Read the model definition and answer for the solid it produces. Units are mm, in the model's axes. Give positions to 0.01 mm unless a question says otherwise; leave off trailing zeros. Order: outer loops, then holes, each group sorted by start corner. A loop starts at its lowest first (then second) coordinate and runs counter-clockwise, first axis right, second up. Notation, with made-up numbers: (-29.75, 46) -> (-20.75, 46) arc R17 cw to (-20.75, 53) -> close; hole circle Ø1 at (29, 69). An arc over 180 degrees is marked (long way). Answer as CSV lines item,"result". Start each with the question number.
1) Find section C-C (y = 225). Determine the outline of the cut face in (x, z), and give its area (3 significant figures).
2) Find section A-A (z = 0). Determine the outline of the cut face in (x, y).
3) Straight lines are drawn through the part: L1, parallel to X at y = 182, z = 0; L2, parallel to Y at x = 52, z = 4; L3, parallel to Y at x = -71.5, z = 43. For each, find the intervals that lie inside material, in ascending order. Write a range as from..to.
4) Flat-ended cylindrical pins translate along their axes: pin 1 Ø5 at (y, z) = (34.5, -28.5) entering from -X; pin 2 Ø2 at (x, y) = (68.5, 104) entering from -Z; pin 3 Ø1.5 at (y, z) = (180.5, 43) entering from -X; pin 4 Ø1 at (x, z) = (-42, -33) entering from -Y. Find the tip coordinate at first contact, or state that the pin passes through.
5) Find section B-B (x = 0). Determine the outline of the cut face in (y, z).
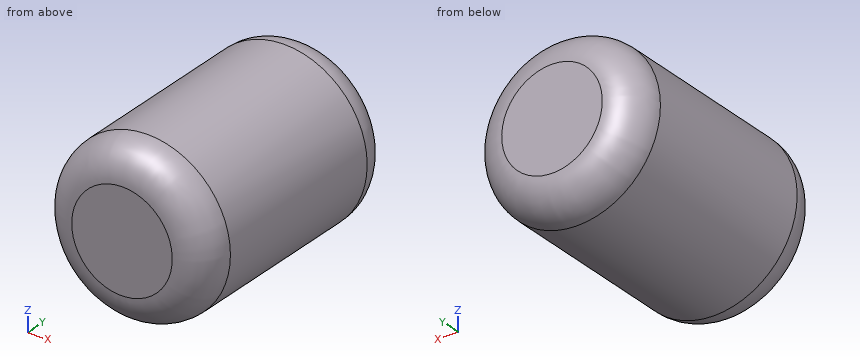
```python
from build123d import *

# Parameters (mm, degrees)
SKETCH1_R           = 100
SKETCH1_R_2         = 98
BOSS_EXTRUDE1_DEPTH = 300
SKETCH2_R           = 100
BOSS_EXTRUDE2_DEPTH = 2
SKETCH4_R           = 100
BOSS_EXTRUDE3_DEPTH = 2
FILLET1_R           = 40


with BuildPart() as part:
    # Sketch1 → Boss-Extrude1 (new body)
    with BuildSketch(Plane(origin=(0, 0, 0), x_dir=(1, 0, 0), z_dir=(0, 1, 0))):
        with Locations(Location((0, 0, 0), (0, 0, 270))):
            Circle(SKETCH1_R)
        with Locations(Location((0, 0, 0), (0, 0, 270))):
            Circle(SKETCH1_R_2, mode=Mode.SUBTRACT)
    extrude(amount=BOSS_EXTRUDE1_DEPTH)

    # Sketch2 → Boss-Extrude2 (add)
    with BuildSketch(Plane.XZ):
        with Locations(Location((0, 0, 0), (0, 0, 90))):
            Circle(SKETCH2_R)
    extrude(amount=-BOSS_EXTRUDE2_DEPTH)

    # Sketch4 → Boss-Extrude3 (add)
    with BuildSketch(Plane(origin=(0, 300, 0), x_dir=(1, 0, 0), z_dir=(0, 1, 0))):
        with Locations(Location((0, 0, 0), (0, 0, 270))):
            Circle(SKETCH4_R)
    extrude(amount=BOSS_EXTRUDE3_DEPTH)

    # Fillet1
    fillet1_edges = [part.edges().sort_by_distance(p)[0] for p in [
        (0, 2, -98),
        (0, 300, -98),
        (0, 302, -100),
        (0, 0, -100),
    ]]
    fillet(fillet1_edges, radius=FILLET1_R)


solid = part.part
```
Findings below:
1,outline,"circle Ø200 at (0, 0); hole circle Ø196 at (0, 0)"
1,area,"1,240 mm²"
2,outline,"(-100, 40) arc R40 ccw to (-60, 0) -> (60, 0) arc R40 ccw to (100, 40) -> (100, 262) arc R40 ccw to (60, 302) -> (-60, 302) arc R40 ccw to (-100, 262) -> close; hole (-98, 42) arc R40 ccw to (-58, 2) -> (58, 2) arc R40 ccw to (98, 42) -> (98, 260) arc R40 ccw to (58, 300) -> (-58, 300) arc R40 ccw to (-98, 260) -> close"
3,L1,"-100..-98, 98..100"
3,L2,"0..2, 300..302"
3,L3,"7.58..11.13, 290.87..294.42"
4,pin 1,"x = -96.24"
4,pin 2,"z = -73.78"
4,pin 3,"x = -90.64"
4,pin 4,"y = 0"
5,outline,"(0, -60) arc R40 ccw to (40, -100) -> (262, -100) arc R40 ccw to (302, -60) -> (302, 60) arc R40 ccw to (262, 100) -> (40, 100) arc R40 ccw to (0, 60) -> close; hole (2, -58) arc R40 ccw to (42, -98) -> (260, -98) arc R40 ccw to (300, -58) -> (300, 58) arc R40 ccw to (260, 98) -> (42, 98) arc R40 ccw to (2, 58) -> close"
